from build123d import *

# Parameters (mm, degrees)
SKETCH3_R          = 0.79375
CUT_EXTRUDE1_DEPTH = 1.5875


with BuildPart() as part:
    # Sketch1 → Revolve1 (revolve)
    with BuildSketch(Plane(origin=(0, 0, 0), x_dir=(0, 0, -1), z_dir=(1, 0, 0)), mode=Mode.PRIVATE) as revolve1_sk:
        with BuildLine():
            Line((-21.59, 0), (-21.59, 26.9875))
            Line((-21.59, 26.9875), (-25.4, 26.9875))
            Line((-25.4, 26.9875), (-25.4, 44.45))
            Line((-25.4, 44.45), (-28.575, 44.45))
            Line((-28.575, 44.45), (-28.575, 39.527129933))
            ThreePointArc((-28.575, 39.527129933), (-29.163802958, 36.527036929), (-30.842857143, 33.972037124))
            ThreePointArc((-30.842857143, 33.972037124), (-31.514478817, 32.950037202), (-31.75, 31.75))
            Line((-31.75, 31.75), (-31.75, 0))
            Line((-31.75, 0), (-21.59, 0))
        make_face()
    revolve(revolve1_sk.sketch.rotate(Axis((0, 0, 31.75), (0, 0, -1)), 90), axis=Axis((0, 0, 31.75), (0, 0, -1)))

    # Sketch2 → Cut-Revolve1 (revolve, cut)
    with BuildSketch(Plane(origin=(0, 0, 0), x_dir=(0, 0, -1), z_dir=(1, 0, 0)), mode=Mode.PRIVATE) as cut_revolve1_sk:
        Polygon((-30.1625, 25.4), (-23.1775, 25.4), (-23.1775, 0), (-31.75, 0), (-31.75, 6.35), (-30.1625, 6.35), align=None)
    revolve(cut_revolve1_sk.sketch.rotate(Axis((0, 0, 31.75), (0, 0, -1)), 180), axis=Axis((0, 0, 31.75), (0, 0, -1)), mode=Mode.SUBTRACT)

    # Sketch3 → Cut-Extrude1 (cut)
    with BuildSketch(Plane(origin=(0, 0, 21.59), x_dir=(-1, 0, 0), z_dir=(0, 0, -1))):
        with Locations((0, 3.175)):
            Circle(SKETCH3_R)
        with Locations((2.749630657, 1.5875)):
            Circle(SKETCH3_R)
        with Locations((2.749630657, -1.5875)):
            Circle(SKETCH3_R)
        with Locations((0, -3.175)):
            Circle(SKETCH3_R)
        with Locations((-2.749630657, -1.5875)):
            Circle(SKETCH3_R)
        with Locations((-2.749630657, 1.5875)):
            Circle(SKETCH3_R)
    extrude(amount=-CUT_EXTRUDE1_DEPTH, mode=Mode.SUBTRACT)


solid = part.part
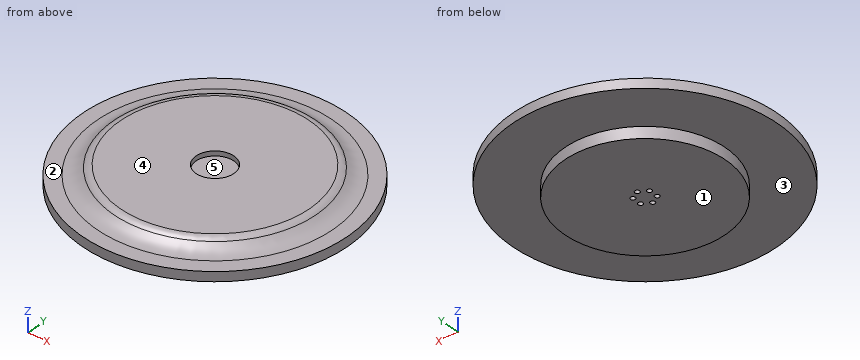
Geometry check sheet. Reference: the model listing, model coordinates, mm. Face numbers are marked on the shaded views. A direction names the side the tool comes from. Round coordinates to 2 decimals unless told otherwise and drop trailing zeros.
Item 1: Thickness scan on line 1 (Y direction, x = 0, z = 22.25); line 2 (Z direction, x = 13, y = 12); line 3 (Z direction, x = -37, y = 22) (3 decimals). Record the ranges inside material, lowest first.
Item 2: Mould release check, pull along Z, two halves, no side actions. Record for the marked faces 3, 4 and 5: pulls with the +Z half, pulls with the -Z half, needs draft (parallel to the pull), parting line crosses it, or undercut.
Item 3: Gauge pin test, flat ends, axial feed: pin 1 (1 mm diameter, centred on x = 8, z = 25, fed in from +Y); pin 2 (1 mm diameter, centred on x = 0, y = 3.175, fed in from -Z); pin 3 (6 mm diameter, centred on y = -29.5, z = 24, fed in from +X); pin 4 (8 mm diameter, centred on x = 16, y = 29.5, fed in from +Z). Record the tip position at first contact, or that the pin passes through.
Item 4: Access from +Z, -Z, +X, -X, +Y, -Y to the whole of each face (thin tool, end or side, straight path). Record for the marked faces 1 and 2.
Answer sheet:
1. line 1: y = -26.99 to -3.97, -2.38 to 2.38, 3.97 to 26.99
1. line 2: z = 21.59 to 23.18, 30.16 to 31.75
1. line 3: z = 25.4 to 28.575
2. face 3: pulls with the -Z half
2. face 4: pulls with the +Z half
2. face 5: undercut
3. pin 1: stops at y = 43.78
3. pin 2: passes through
3. pin 3: stops at x = 35.43
3. pin 4: stops at z = 31.75
4. face 1: -Z, +X, -X, +Y, -Y
4. face 2: +Z
